from build123d import *

# Parameters (mm, degrees)
SKETCH_1_W      = 80
SKETCH_1_H      = 62
SKETCH_1_R      = 1.6
SKETCH_1_R_2    = 11.25
EXTRUDE_1_DEPTH = 3


with BuildPart() as part:
    # 草图1 → 凸台-拉伸1 (new body)
    with BuildSketch(Plane(origin=(0, 0, 0), x_dir=(1, 0, 0), z_dir=(0, 1, 0))):
        with Locations((40, -31)):
            Rectangle(SKETCH_1_W, SKETCH_1_H)
        with Locations(Location((10, -10, 0), (0, 0, 270))):
            Circle(SKETCH_1_R, mode=Mode.SUBTRACT)
        with Locations(Location((10, -30, 0), (0, 0, 270))):
            Circle(SKETCH_1_R, mode=Mode.SUBTRACT)
        with Locations(Location((10, -45, 0), (0, 0, 270))):
            Circle(SKETCH_1_R, mode=Mode.SUBTRACT)
        with Locations(Location((10, -60, 0), (0, 0, 270))):
            Circle(SKETCH_1_R, mode=Mode.SUBTRACT)
        with Locations(Location((30, -10, 0), (0, 0, 270))):
            Circle(SKETCH_1_R, mode=Mode.SUBTRACT)
        with Locations(Location((71, -25, 0), (0, 0, 270))):
            Circle(SKETCH_1_R, mode=Mode.SUBTRACT)
        with Locations(Location((40, -25, 0), (0, 0, 270))):
            Circle(SKETCH_1_R, mode=Mode.SUBTRACT)
        with Locations(Location((40, -56, 0), (0, 0, 270))):
            Circle(SKETCH_1_R, mode=Mode.SUBTRACT)
        with Locations(Location((71, -56, 0), (0, 0, 270))):
            Circle(SKETCH_1_R, mode=Mode.SUBTRACT)
        with Locations(Location((55.5, -40.5, 0), (0, 0, 270))):
            Circle(SKETCH_1_R_2, mode=Mode.SUBTRACT)
        with Locations(Location((50, -10, 0), (0, 0, 270))):
            Circle(SKETCH_1_R, mode=Mode.SUBTRACT)
        with Locations(Location((70, -10, 0), (0, 0, 270))):
            Circle(SKETCH_1_R, mode=Mode.SUBTRACT)
        with Locations(Location((31.5, -30, 0), (0, 0, 270))):
            Circle(SKETCH_1_R, mode=Mode.SUBTRACT)
        with Locations(Location((31.5, -45, 0), (0, 0, 270))):
            Circle(SKETCH_1_R, mode=Mode.SUBTRACT)
    extrude(amount=EXTRUDE_1_DEPTH)


solid = part.part
Input: part model. Units: mm. Frame: model coordinates. Coordinates: 2 decimals unless noted, no trailing zeros. Order: outer loops, then holes, each group sorted by start corner. A loop starts at its lowest first (then second) coordinate and runs counter-clockwise, first axis right, second up. Notation, with made-up numbers: M 63.5,-16 L 83.5,-16 A22 cw 83.5,14 Z; hole C -11,10 d8. An arc over 180 degrees is marked long. Answer as CSV lines item,"result".
1. Material intervals for line 1 (X direction, y = 1.5, z = 56); line 2 (Z direction, x = 70, y = 1.15); line 3 (X direction, y = 1.1, z = 10), sorted ascending. Write a range as from..to.
Reported:
line 1,"0..38.4, 41.6..69.4, 72.6..80"
line 2,"0..8.4, 11.6..23.75, 26.25..54.75, 57.25..62"
line 3,"0..8.4, 11.6..28.4, 31.6..48.4, 51.6..68.4, 71.6..80"
2. Section A-A (z = 40.5). Return the cut outline in (x, y).
Reported:
outline,"M 0,0 L 44.25,0 L 44.25,3 L 0,3 Z; M 66.75,0 L 80,0 L 80,3 L 66.75,3 Z"
3. Section C-C (z = 56). Return the cut outline in (x, y), then the cut area to 3 significant figures.
Reported:
outline,"M 0,0 L 38.4,0 L 38.4,3 L 0,3 Z; M 41.6,0 L 69.4,0 L 69.4,3 L 41.6,3 Z; M 72.6,0 L 80,0 L 80,3 L 72.6,3 Z"
area,"221 mm2"
4. Section D-D (z = 49). Return the cut outline in (x, y), then the cut area to 3 significant figures.
Reported:
outline,"M 0,0 L 48.13,0 L 48.13,3 L 0,3 Z; M 62.87,0 L 80,0 L 80,3 L 62.87,3 Z"
area,"196 mm2"
5. Pull-direction query (X, two-part tool) for faces 1 (the cylindrical face through (8.44, 1.48, 44.65)), 2 (the flat face through (80, 1, 31)), 3 (the flat face through (39, 3, 31)), 4 (the flat face through (0, 1, 31)); classes: released by +X, released by -X, zero draft, split by the parting line, or undercut.
Reported:
face 1,"undercut"
face 2,"released by +X"
face 3,"zero draft"
face 4,"released by -X"
6. Section B-B (y = 2.2). State how many separate pieces and enclosed holes the cut face has, then the cut area to 3 significant figures.
Reported:
separate pieces,"1"
enclosed holes,"14"
area,"4,460 mm2"
